```python
from build123d import *

# Parameters (mm, degrees)
BASPROSKE_W        = 10
BASPROSKE_H        = 16
TOOTHCUT_DEPTH     = 25.738633754
TEETHCUTS_COUNT    = 14
TEETHCUTS_ANGLE    = 334.285714286
BORSKE_R           = 3
BORE_DEPTH         = 50.0000508
HOLE_WIZARD_M3_1_D = 3.5


with BuildPart() as part:
    # BasProSke → Base-Revolve (revolve)
    with BuildSketch(Plane(origin=(0, 0, 0), x_dir=(1, 0, 0), z_dir=(0, 1, 0)), mode=Mode.PRIVATE) as base_revolve_sk:
        with Locations((5, 8)):
            Rectangle(BASPROSKE_W, BASPROSKE_H)
    revolve(base_revolve_sk.sketch.rotate(Axis((-10, 0, 0), (1, 0, 0)), 180), axis=Axis((-10, 0, 0), (1, 0, 0)))

    # TooCutSke → ToothCut (cut, through all)
    with BuildSketch(Plane(origin=(0, 0, 0), x_dir=(0, 0, -1), z_dir=(1, 0, 0))):
        with BuildLine():
            ThreePointArc((1.067858192, 11.449309144), (0, 11.499), (-1.067858192, 11.449309144))
            ThreePointArc((-1.067858192, 11.449309144), (-1.641684211, 13.812780716), (-3.163375005, 15.710076503))
            ThreePointArc((-3.163375005, 15.710076503), (0, 16.0254), (3.163375005, 15.710076503))
            ThreePointArc((3.163375005, 15.710076503), (1.641684211, 13.812780716), (1.067858192, 11.449309144))
        make_face()
    toothcut = extrude(amount=TOOTHCUT_DEPTH, mode=Mode.SUBTRACT)

    # TeethCuts: ToothCut ×14 about axis
    teethcuts_axis = Axis((-10, 0, 0), (1, 0, 0))
    for i in range(1, TEETHCUTS_COUNT):
        add(toothcut.rotate(teethcuts_axis, i * TEETHCUTS_ANGLE / (TEETHCUTS_COUNT - 1)), mode=Mode.SUBTRACT)

    # BorSke → Bore (cut, symmetric)
    with BuildSketch(Plane(origin=(0, 0, 0), x_dir=(0, 0, -1), z_dir=(1, 0, 0))):
        with Locations(Location((0, 0, 0), (0, 0, 180))):
            Circle(BORSKE_R)
    extrude(amount=BORE_DEPTH, both=True, mode=Mode.SUBTRACT)

    # M3 すきま穴1 (through all)
    with Locations(Plane.ZY):
        with Locations((7.5, 0), (-7.5, 0)):
            Hole(HOLE_WIZARD_M3_1_D / 2)


solid = part.part
```
CAD build for the part. Positions are in the model's coordinates, mm. A direction names the side the tool comes from. Coordinates: 2 decimals unless noted, no trailing zeros. Write each loop counter-clockwise with the first axis right and the second up, starting at its lowest first coordinate (ties: lowest second). Pieces come first, ordered by that corner, then holes.
(1) Drill centre lines: probe 1 along Y at (x, z) = (6.25, 0); probe 2 along Y at (x, z) = (2.25, 14); probe 3 along Z at (x, y) = (3.5, 12). Where is each one in solid material? Low to high.
(2) Cut at B-B, the plane y = 0. List the corners of the cut face in (x, z), and give its area (3 significant figures).
(3) 3-axis set-ups, long thin cutter, end or side, ignore diameter. For faces 5 (the face through (5.07, -15.597, 3.566)), 6 (the face through (4.93, 7.318, 11.773)), 7 (the face through (4.93, -9.912, -9.783)), 8 (the face through (4.93, 9.912, 9.783)): which of +Z, -Z, +X, -X, +Y, -Y reach the whole face in a straight line?
(4) Two-plate mould, pull along Y, no slides. Class faces 1 (the face through (4.93, 13.83, -1.65)), 2 (the face through (4.93, -10.367, -4.976)), 3 (the face through (5.07, 0.526, 5.831)), 4 (the face through (4.93, -13.77, -1.62)): +Y half, -Y half, draft (parallel to the pull), parting line (faces both ways), or undercut.
(5) Cut at A-A, the plane z = 0. List the corners of the cut face in (x, y).
(6) Cut at C-C, the plane z = -7.5. List the corners of the cut face in (x, y).
(7) Flat gauge pins, fed straight in: pin 1 (1 mm diameter, centred on y = -6, z = -10, fed in from -X); pin 2 (1 mm diameter, centred on x = 4.5, y = 12.5, fed in from -Z); pin 3 (1 mm diameter, centred on x = 8, z = 11, fed in from -Y); pin 4 (1.5 mm diameter, centred on x = 5, y = -9, fed in from -Z). Where does each tip first touch, or does it go through?
(8) Cut at D-D, the plane x = 2.5. Count the separate pieces of the cut face and the enclosed holes in it, and give its area (3 significant figures).
Geometry says:
1. probe 1: y = -11.5 to -3, 3 to 11.5
1. probe 2: y = -7.37 to -5.59, -1.43 to 1.43, 5.59 to 7.37
1. probe 3: z = -10.3 to -7.84, -4.4 to -1.11, 1.11 to 4.4, 7.84 to 10.3
2. outline: (0, -16) - (10, -16) - (10, -9.25) - (0, -9.25) - close; (0, -5.75) - (10, -5.75) - (10, -3) - (0, -3) - close; (0, 3) - (10, 3) - (10, 5.75) - (0, 5.75) - close; (0, 9.25) - (10, 9.25) - (10, 16) - (0, 16) - close
2. area: 190 mm2
3. face 5: +Z, +X, -X, -Y
3. face 6: +X, -X
3. face 7: -Z, +X, -X
3. face 8: +Z, +X, -X
4. face 1: +Y half
4. face 2: undercut
4. face 3: undercut
4. face 4: -Y half
5. outline: (0, -11.5) - (10, -11.5) - (10, -3) - (0, -3) - close; (0, 3) - (10, 3) - (10, 11.5) - (0, 11.5) - close
6. outline: (0, -11.75) - (10, -11.75) - (10, -1.75) - (0, -1.75) - close; (0, 1.75) - (10, 1.75) - (10, 11.75) - (0, 11.75) - close
7. pin 1: stops at x = 0
7. pin 2: stops at z = -10.31
7. pin 3: stops at y = -7.25
7. pin 4: stops at z = -9.7
8. separate pieces: 1
8. enclosed holes: 3
8. area: 536 mm2
